```python
from build123d import *

# Parameters (mm, degrees)
ESQUISSE2_W             = 53.3
ESQUISSE2_H             = 20
BOSS_EXTRU_1_DEPTH      = 15
CONG_1_R                = 3
ESQUISSE4_W             = 20
ESQUISSE4_H             = 10
ENL_V_MAT_EXTRU_1_DEPTH = 31
ESQUISSE5_R             = 2.5
ENL_V_MAT_EXTRU_2_DEPTH = 21


with BuildPart() as part:
    # Esquisse2 → Boss.-Extru.1 (new body, symmetric)
    with BuildSketch(Plane(origin=(0, 0, 0), x_dir=(1, 0, 0), z_dir=(0, 1, 0))):
        with Locations((26.65, 0)):
            Rectangle(ESQUISSE2_W, ESQUISSE2_H)
    extrude(amount=BOSS_EXTRU_1_DEPTH, both=True)

    # Congé1
    cong_1_edges = [part.edges().sort_by_distance(p)[0] for p in [
        (53.3, 15, 0),
        (0, 15, 0),
        (53.3, -15, 0),
        (0, -15, 0),
    ]]
    fillet(cong_1_edges, radius=CONG_1_R)

    # Esquisse4 → Enlèv. mat.-Extru.1 (cut, through all)
    with BuildSketch(Plane(origin=(0, 15, 0), x_dir=(1, 0, 0), z_dir=(0, 1, 0))):
        with Locations((43.3, 0)):
            Rectangle(ESQUISSE4_W, ESQUISSE4_H)
    extrude(amount=-ENL_V_MAT_EXTRU_1_DEPTH, mode=Mode.SUBTRACT)

    # Esquisse5 → Enlèv. mat.-Extru.2 (cut, through all)
    with BuildSketch(Plane(origin=(0, 0, -10), x_dir=(-1, 0, 0), z_dir=(0, 0, -1))):
        with Locations((-48.3, 10)):
            Circle(ESQUISSE5_R)
        with Locations((-5, 10)):
            Circle(ESQUISSE5_R)
    extrude(amount=-ENL_V_MAT_EXTRU_2_DEPTH, mode=Mode.SUBTRACT)


solid = part.part
```
CAD build for the part. Positions are in the model's coordinates, mm. A direction names the side the tool comes from. Give positions to 0.01 mm unless a question says otherwise; leave off trailing zeros. Write each loop counter-clockwise with the first axis right and the second up, starting at its lowest first coordinate (ties: lowest second). Pieces come first, ordered by that corner, then holes. Notation, with made-up numbers: M 16.25,30.25 L 55.25,30.25 A27 ccw 55.25,62.25 Z; hole C 20,2 d2. An arc over 180 degrees is marked long. Return JSON: item names as keys, results as strings. Group by question number.
(1) Drill centre lines: L1, parallel to Z at x = 51, y = 1.5; L2, parallel to Y at x = 48.3, z = 8.05; L3, parallel to X at y = 0.5, z = -1.75. Where is each one in solid material? Low to high. Write a range as [from, to].
(2) Band-saw the part on A-A (y = 10). Give the cut face in (x, z), and give its area (3 significant figures).
(3) Band-saw the part on D-D (x = 36). Give the cut face in (y, z).
(4) Band-saw the part on C-C (x = 48.3). Give the cut face in (y, z).
(5) Mould opens along X. For faces 1 (the face through (43, 0, 5)), 2 (the face through (53.3, 0, 8)), 3 (the face through (50.8, 10.1, 7.5)), 4 (the face through (0, 0, 0)) say: pulls with the +X half, pulls with the -X half, needs draft (parallel to the pull), parting line crosses it, or undercut.
(6) 3-axis set-ups, long thin cutter, end or side, ignore diameter. For faces 5 (the face through (33.3, 0, 0)), 6 (the face through (26, 0, -10)): which of +Z, -Z, +X, -X, +Y, -Y reach the whole face in a straight line?
(7) Band-saw the part on B-B (z = -6.5). Give the cut face in (x, y), and give its area (3 significant figures).
(8) Flat gauge pins, fed straight in: pin 1 Ø11 at (y, z) = (6, 1) entering from +X; pin 2 Ø2 at (y, z) = (0.5, -2.5) entering from +X. Where does each tip first touch, or does it go through?
Entries:
{
 "1": {"L1": "z = [-10, -5], [5, 10]", "L2": "y = [-15, 7.5], [12.5, 15]", "L3": "x = [0, 33.3]"},
 "2": {"outline": "M 0,-10 L 2.5,-10 L 2.5,10 L 0,10 Z; M 7.5,-10 L 45.8,-10 L 45.8,-5 L 33.3,-5 L 33.3,5 L 45.8,5 L 45.8,10 L 7.5,10 Z; M 50.8,-10 L 53.3,-10 L 53.3,-5 L 50.8,-5 Z; M 50.8,5 L 53.3,5 L 53.3,10 L 50.8,10 Z", "area": "716 mm^2"},
 "3": {"outline": "M -15,-10 L 15,-10 L 15,-5 L -15,-5 Z; M -15,5 L 15,5 L 15,10 L -15,10 Z"},
 "4": {"outline": "M -15,-10 L 7.5,-10 L 7.5,-5 L -15,-5 Z; M -15,5 L 7.5,5 L 7.5,10 L -15,10 Z; M 12.5,-10 L 15,-10 L 15,-5 L 12.5,-5 Z; M 12.5,5 L 15,5 L 15,10 L 12.5,10 Z"},
 "5": {"face 1": "needs draft", "face 2": "pulls with the +X half", "face 3": "undercut", "face 4": "pulls with the -X half"},
 "6": {"face 5": "+X, +Y, -Y", "face 6": "-Z, +X, -X, +Y, -Y"},
 "7": {"outline": "M 0,-12 A3 ccw 3,-15 L 50.3,-15 A3 ccw 53.3,-12 L 53.3,12 A3 ccw 50.3,15 L 3,15 A3 ccw 0,12 Z; hole C 5,10 d5; hole C 48.3,10 d5", "area": "1,550 mm^2"},
 "8": {"pin 1": "stops at x = 53.3", "pin 2": "stops at x = 33.3"}
}
